Drawing for the job (mm, zero at the part's lowest x, y, z). A direction names the side the tool comes from. Give positions to 0.01 mm unless a question says otherwise; leave off trailing zeros. Loops run counter-clockwise (first coordinate to the right, second up) from the corner with the lowest first, then second, coordinate; pieces in that order, holes last. Notation, with made-up numbers: (-31, 67) -> (-11, 67) arc R25 ccw to (-11, 95) -> close; hole circle Ø1 at (66, 69). An arc over 180 degrees is marked (long way). Use CSV: the item, a comma, the result in double quotes. Start each with the question number.
(1) 3-axis set-ups, long thin cutter, end or side, ignore diameter. For the marked faces 4, 5 and 6: which of +Z, -Z, +X, -X, +Y, -Y reach the whole face in a straight line?
(2) Cut at D-D on y = 12.5. Write the cut outline in (x, z).
(3) Drill centre lines: probe 1 along Z at (x, y) = (18.5, 4.5); probe 2 along Z at (x, y) = (18, 19.25). Where is each one in solid material? Low to high.
(4) Pull direction Z, two halves, no side cores. Call the marked faces 1, 2 and 3: pulls with the +Z half, pulls with the -Z half, needs draft (parallel to the pull), parting line crosses it, or undercut.
(5) Cut at C-C on z = 9.25. Write the cut outline in (x, y).
(6) Cut at B-B on x = 7. Write the cut outline in (y, z), then the cut area to 3 significant figures.
(7) Flat gauge pins, fed straight in: pin 1 (8 mm diameter, centred on x = 2.5, y = 12.5, fed in from +Z); pin 2 (1.6 mm diameter, centred on x = 14, z = 9, fed in from +Y); pin 3 (1 mm diameter, centred on x = 17, y = 19, fed in from +Z). Where does each tip first touch, or does it go through?
(8) Cut at A-A on y = 7.75. Write the cut outline in (x, z), then the cut area to 3 significant figures.
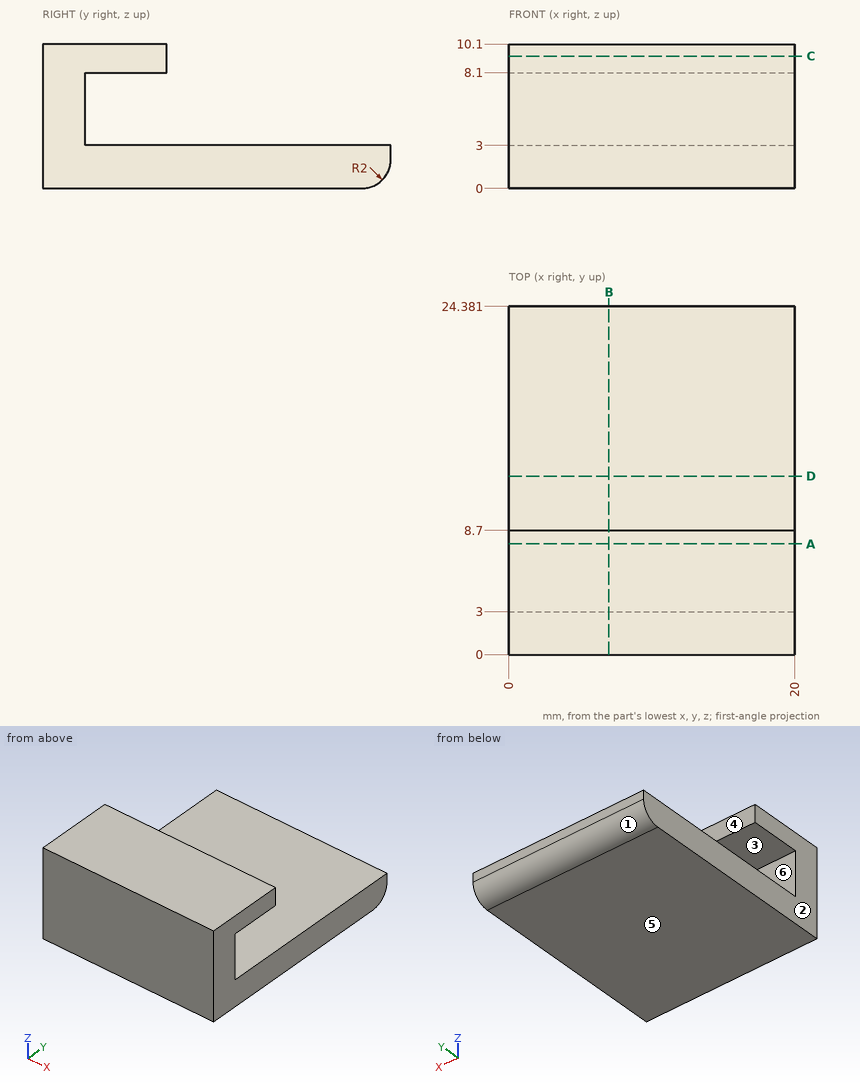
Check result:
1,face 4,"+Z, +X, -X, +Y"
1,face 5,"-Z, +X, -X, +Y, -Y"
1,face 6,"+X, -X, +Y"
2,outline,"(0, 0) -> (20, 0) -> (20, 3) -> (0, 3) -> close"
3,probe 1,"0 to 3, 8.1 to 10.1"
3,probe 2,"0 to 3"
4,face 1,"pulls with the -Z half"
4,face 2,"needs draft"
4,face 3,"undercut"
5,outline,"(0, 0) -> (20, 0) -> (20, 8.7) -> (0, 8.7) -> close"
6,outline,"(0, 0) -> (22.38, 0) arc R2 ccw to (24.38, 2) -> (24.38, 3) -> (3, 3) -> (3, 8.1) -> (8.7, 8.1) -> (8.7, 10.1) -> (0, 10.1) -> close"
6,area,"105 mm²"
7,pin 1,"z = 10.1"
7,pin 2,"y = 8.7"
7,pin 3,"z = 3"
8,outline,"(0, 0) -> (20, 0) -> (20, 3) -> (0, 3) -> close; (0, 8.1) -> (20, 8.1) -> (20, 10.1) -> (0, 10.1) -> close"
8,area,"100 mm²"
